Autodesk Inventor part; units mm, degrees
ref_plane "YZ Plane" through (0, 0, 0) normal (1, 0, 0) x (0, 1, 0)
ref_plane "XZ Plane" through (0, 0, 0) normal (0, 1, 0) x (-1, 0, 0)
ref_plane "XY Plane" through (0, 0, 0) normal (0, 0, 1) x (1, 0, 0)
sketch "スケッチ1" plane through (0, 0, 0) normal (0, 0, 1) x (1, 0, 0)
  circle A0 centre (0, 0) radius 40.5
  dimension "d0" = 81
extrude "プレート1" add sketch "スケッチ1" along normal mid plane 1
sketch "スケッチ2" plane through (0, 0, 0.5) normal (0, 0, 1) x (1, 0, 0)
  circle A0 centre (0, 0) radius 12.05
  dimension "d2" = 24.1
extrude "押し出し1" cut sketch "スケッチ2" against normal blind 10
sketch "スケッチ3" plane through (0, 0, 0.5) normal (0, 0, 1) x (1, 0, 0)
  circle A0 centre (0, 0) radius 32
  point P0 (0, 32)
  point P1 (-27.7128, 16)
  point P2 (-27.7128, -16)
  point P3 (0, -32)
  point P4 (27.7128, -16)
  point P5 (27.7128, 16)
  dimension "d5" = 64
  dimension "d8" = 360
hole "穴1" at (0, 32, 0.5) at (-27.7128, 16, 0.5) at (-27.7128, -16, 0.5) at (0, -32, 0.5) at (27.7128, -16, 0.5) at (27.7128, 16, 0.5) direction (0, 0, -1) diameter 4.3 end through all
equation "\"d15\" = Thickness"
equation "\"d1\" = Thickness"
equation "\"BendRadius\" = Thickness"
equation "\"BendReliefWidth\" = Thickness"
equation "\"BendReliefDepth\" = 0.5 * Thickness"
equation "\"CornerReliefSize\" = 4 * Thickness"
equation "\"MinimumRemnant\" = 2 * Thickness"
equation "\"TransitionRadius\" = BendRadius"
equation "\"JacobiRadiusSize\" = BendRadius"
equation "\"GapSize\" = Thickness"
properties part number "unit-plate1" material "CFRP"
The listing builds one solid part. Answer for the finished solid, in the listing's coordinates (mm). Round coordinates to 2 decimals unless told otherwise and drop trailing zeros. Order: outer loops, then holes, each group sorted by start corner. A loop starts at its lowest first (then second) coordinate and runs counter-clockwise, first axis right, second up. Notation, with made-up numbers: (-9, 12) - (47, 12) arc R22 ccw to (47, 42) - close; hole circle Ø10 at (89.5, 47). An arc over 180 degrees is marked (long way). Write item = value, one per line. Start each with the question number.
1) Section B-B, the plane y = 16 is taken. Write down the section's boundary in (x, z).
2) Section C-C, the plane z = -0.15 is taken. Write down the section's boundary in (x, y).
3) For a pull along X with two mould halves and no side action, classify faces 1 (the cylindrical face through (-0.65, 29.95, -0.01)), 2 (the cylindrical face through (21.77, -34.15, -0.01)), 3 (the flat face through (8, 10, -0.5)) as released by +X, released by -X, zero draft, split by the parting line, or undercut.
4) Section D-D, the plane y = 32 is taken. Write down the section's boundary in (x, z), plus the area to 3 significant figures.
5) Section A-A, the plane x = 0 is taken. Write down the section's boundary in (y, z), plus the area to 3 significant figures.
6) Straight lines are drawn through the part: L1, parallel to Y at x = 0, z = -0.2; L2, parallel to X at y = 0.5, z = 0.4; L3, parallel to Y at x = -27, z = 0.1. For each, find the intervals that lie inside material, in ascending order.
Results list:
q1.outline = (-37.21, -0.5) - (-29.86, -0.5) - (-29.86, 0.5) - (-37.21, 0.5) - close; (-25.56, -0.5) - (25.56, -0.5) - (25.56, 0.5) - (-25.56, 0.5) - close; (29.86, -0.5) - (37.21, -0.5) - (37.21, 0.5) - (29.86, 0.5) - close
q2.outline = circle Ø81 at (0, 0); hole circle Ø4.3 at (-27.71, -16); hole circle Ø4.3 at (-27.71, 16); hole circle Ø24.1 at (0, 0); hole circle Ø4.3 at (0, -32); hole circle Ø4.3 at (0, 32); hole circle Ø4.3 at (27.71, -16); hole circle Ø4.3 at (27.71, 16)
q3.face_1 = undercut
q3.face_2 = split by the parting line
q3.face_3 = zero draft
q4.outline = (-24.82, -0.5) - (-2.15, -0.5) - (-2.15, 0.5) - (-24.82, 0.5) - close; (2.15, -0.5) - (24.82, -0.5) - (24.82, 0.5) - (2.15, 0.5) - close
q4.area = 45.3 mm^2
q5.outline = (-40.5, -0.5) - (-34.15, -0.5) - (-34.15, 0.5) - (-40.5, 0.5) - close; (-29.85, -0.5) - (-12.05, -0.5) - (-12.05, 0.5) - (-29.85, 0.5) - close; (12.05, -0.5) - (29.85, -0.5) - (29.85, 0.5) - (12.05, 0.5) - close; (34.15, -0.5) - (40.5, -0.5) - (40.5, 0.5) - (34.15, 0.5) - close
q5.area = 48.3 mm^2
q6.L1 = -40.5 to -34.15, -29.85 to -12.05, 12.05 to 29.85, 34.15 to 40.5
q6.L2 = -40.5 to -12.04, 12.04 to 40.5
q6.L3 = -30.19 to -18.03, -13.97 to 13.97, 18.03 to 30.19
